```python
from build123d import *

# Parameters (mm, degrees)
SKETCH1_W           = 48
SKETCH1_H           = 28
SKETCH1_W_2         = 40
SKETCH1_H_2         = 20
BOSS_EXTRUDE1_DEPTH = 95
SKETCH2_W           = 2.5
SKETCH2_H           = 5
CUT_EXTRUDE1_DEPTH  = 5
SKETCH6_W           = 2.5
SKETCH6_H           = 5
BOSS_EXTRUDE3_DEPTH = 5


with BuildPart() as part:
    # Sketch1 → Boss-Extrude1 (new body)
    with BuildSketch(Plane(origin=(0, 0, 0), x_dir=(1, 0, 0), z_dir=(0, 1, 0))):
        with Locations((20, -10)):
            Rectangle(SKETCH1_W, SKETCH1_H)
        with Locations((20, -10)):
            Rectangle(SKETCH1_W_2, SKETCH1_H_2, mode=Mode.SUBTRACT)
    extrude(amount=BOSS_EXTRUDE1_DEPTH)

    # Sketch2 → Cut-Extrude1 (cut)
    with BuildSketch(Plane(origin=(0, 95, 0), x_dir=(1, 0, 0), z_dir=(0, 1, 0))):
        with Locations((-2.75, -10)):
            Rectangle(SKETCH2_W, SKETCH2_H)
        with Locations((42.75, -10)):
            Rectangle(SKETCH2_W, SKETCH2_H)
    extrude(amount=-CUT_EXTRUDE1_DEPTH, mode=Mode.SUBTRACT)

    # Sketch6 → Boss-Extrude3 (add)
    with BuildSketch(Plane.XZ):
        with Locations((-2.75, 10)):
            Rectangle(SKETCH6_W, SKETCH6_H)
        with Locations((42.75, 10)):
            Rectangle(SKETCH6_W, SKETCH6_H)
    extrude(amount=BOSS_EXTRUDE3_DEPTH)


solid = part.part
```
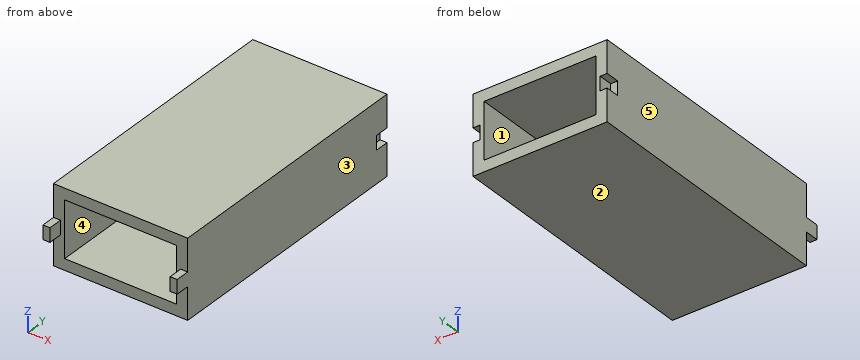
Work out the finished part from the listing and answer in its coordinate system (mm). Face numbers are marked on the shaded views. A direction names the side the tool comes from. Coordinates: 2 decimals unless noted, no trailing zeros. Order: outer loops, then holes, each group sorted by start corner. A loop starts at its lowest first (then second) coordinate and runs counter-clockwise, first axis right, second up. Notation, with made-up numbers: (60, 5) - (80, 5) arc R11 cw to (80, 16) - close; hole circle Ø4 at (-15, -3.75). An arc over 180 degrees is marked (long way). Answer as a JSON object with one key per item and string values.
1. Find section C-C on y = 18. Determine the outline of the cut face in (x, z).
Output values:
{"outline": "(-4, -4) - (44, -4) - (44, 24) - (-4, 24) - close; hole (0, 0) - (40, 0) - (40, 20) - (0, 20) - close"}
2. Find section A-A on x = 15. Determine the outline of the cut face in (y, z), plus the area to 3 significant figures.
Output values:
{"outline": "(0, -4) - (95, -4) - (95, 0) - (0, 0) - close; (0, 20) - (95, 20) - (95, 24) - (0, 24) - close", "area": "760 mm²"}
3. Find section B-B on z = 6.5. Determine the outline of the cut face in (x, y).
Output values:
{"outline": "(-4, 0) - (0, 0) - (0, 95) - (-4, 95) - close; (40, 0) - (44, 0) - (44, 95) - (40, 95) - close"}
4. Each of these flat-tipped pins is pushed along its axis until it touches: P1, Ø4, axis at x = 11, z = 18.5, coming from the -Y side; P2, Ø1.2, axis at x = 42.5, z = 10, coming from the +Y side; P3, Ø2, axis at x = 43, y = -3.5, coming from the -Z side; P4, Ø5, axis at x = 36, z = 7, coming from the +Y side. Where does it stop, or does it pass through?
Output values:
{"P1": "stops at y = 0", "P2": "stops at y = 90", "P3": "stops at z = 7.5", "P4": "passes through"}
5. Find section D-D on z = 21.25. Determine the outline of the cut face in (x, y), plus the area to 3 significant figures.
Output values:
{"outline": "(-4, 0) - (44, 0) - (44, 95) - (-4, 95) - close", "area": "4,560 mm²"}
6. Consider line 1 (X direction, y = 56.5, z = 8); line 2 (Z direction, x = 12.5, y = 21); line 3 (Y direction, x = 18, z = -2). Determine where each line is inside the solid, lowest interval first.
Output values:
{"line 1": "x = -4 to 0, 40 to 44", "line 2": "z = -4 to 0, 20 to 24", "line 3": "y = 0 to 95"}
7. The mould has two halves that part along Z. Classify the marked faces 1, 2 and 3: +Z half, -Z half, draft (parallel to the pull), parting line (faces both ways), or undercut.
Output values:
{"face 1": "undercut", "face 2": "-Z half", "face 3": "draft"}
8. A tool of negligible diameter and unlimited length cuts with its end or side. For the marked faces 4 and 5, from which of +Z, -Z, +X, -X, +Y, -Y can it reach the whole face along a straight path? Write none if from no direction.
Output values:
{"face 4": "+Y, -Y", "face 5": "+Z, -Z, -X, +Y, -Y"}
